The listing builds one solid part. Answer for the finished solid, in the listing's coordinates (mm). Coordinates: 2 decimals unless noted, no trailing zeros. Write each loop counter-clockwise with the first axis right and the second up, starting at its lowest first coordinate (ties: lowest second). Pieces come first, ordered by that corner, then holes.
from build123d import *

# Parameters (mm, degrees)
BOSS_EXTRUDE1_DEPTH = 3.175
SKETCH2_R           = 3.175
CUT_EXTRUDE1_DEPTH  = 3.175


with BuildPart() as part:
    # Sketch1 → Boss-Extrude1 (new body)
    with BuildSketch(Plane(origin=(0, 0, 0), x_dir=(0, 0, -1), z_dir=(1, 0, 0))):
        Polygon((0, 0), (25.4, 0), (50.8, 0), (50.8, 38.1), (25.4, 38.1), (25.4, 264.16), (0, 264.16), align=None)
    extrude(amount=BOSS_EXTRUDE1_DEPTH)

    # Sketch2 → Cut-Extrude1 (cut)
    with BuildSketch(Plane(origin=(3.175, 0, 0), x_dir=(0, 0, -1), z_dir=(1, 0, 0))):
        with Locations((12.7, 247.65)):
            Circle(SKETCH2_R)
        with Locations((38.1, 32)):
            Circle(SKETCH2_R)
        with Locations((12.7, 32)):
            Circle(SKETCH2_R)
    extrude(amount=-CUT_EXTRUDE1_DEPTH, mode=Mode.SUBTRACT)


solid = part.part
1. Section B-B on y = 32 is taken. Give the vertices of the cut face in (x, z) (3 decimals), then the cut area to 3 significant figures.
Results found:
outline: (0, -50.8) - (3.175, -50.8) - (3.175, -41.275) - (0, -41.275) - close; (0, -34.925) - (3.175, -34.925) - (3.175, -15.875) - (0, -15.875) - close; (0, -9.525) - (3.175, -9.525) - (3.175, 0) - (0, 0) - close
area: 121 mm2
2. Section A-A on z = -38.1 is taken. Give the vertices of the cut face in (x, y) (3 decimals).
Results found:
outline: (0, 0) - (3.175, 0) - (3.175, 28.825) - (0, 28.825) - close; (0, 35.175) - (3.175, 35.175) - (3.175, 38.1) - (0, 38.1) - close
3. Flat-ended cylindrical pins translate along their axes: P1, Ø1, axis at x = 2.5, z = -35, coming from the +Y side; P2, Ø4, axis at y = 247.65, z = -12.7, coming from the -X side. Find the tip coordinate at first contact, or state that the pin passes through.
Results found:
P1: stops at y = 38.1
P2: passes through
4. For a pull along Y with two mould halves and no side action, classify faces 1 (the cylindrical face through (1.61, 28.9, -37.41)), 2 (the flat face through (0, 134, -14)) as pulls with the +Y half, pulls with the -Y half, needs draft (parallel to the pull), parting line crosses it, or undercut.
Results found:
face 1: undercut
face 2: needs draft
5. Section D-D on y = 247.65 is taken. Give the vertices of the cut face in (x, z) (3 decimals), then the cut area to 3 significant figures.
Results found:
outline: (0, -25.4) - (3.175, -25.4) - (3.175, -15.875) - (0, -15.875) - close; (0, -9.525) - (3.175, -9.525) - (3.175, 0) - (0, 0) - close
area: 60.5 mm2
6. Find the intervals of material crossed by L1, parallel to Y at x = 1.7, z = -12.7 (3 decimals); L2, parallel to Y at x = 2.4, z = -38.1 (3 decimals); L3, parallel to Z at x = 1.65, y = 247.65 (3 decimals), in increasing order.
Results found:
L1: y = 0 to 28.825, 35.175 to 244.475, 250.825 to 264.16
L2: y = 0 to 28.825, 35.175 to 38.1
L3: z = -25.4 to -15.875, -9.525 to 0
7. Section C-C on x = 0.5 is taken. Give the vertices of the cut face in (y, z) (3 decimals), then the cut area to 3 significant figures.
Results found:
outline: (0, -50.8) - (38.1, -50.8) - (38.1, -25.4) - (264.16, -25.4) - (264.16, 0) - (0, 0) - close; hole circle Ø6.35 at (32, -38.1); hole circle Ø6.35 at (32, -12.7); hole circle Ø6.35 at (247.65, -12.7)
area: 7,580 mm2
